```python
from build123d import *


with BuildPart() as part:
    # Croquis1 → Revolución1 (revolve)
    with BuildSketch(Plane.XY):
        with BuildLine():
            Line((5, 0), (15, 0))
            ThreePointArc((15, 0), (17.5, 2.5), (15, 5))
            Line((15, 5), (17, 9.999396685))
            ThreePointArc((17, 9.999396685), (25.700254064, 18.050962315), (18.873239437, 27.741885964))
            ThreePointArc((18.873239437, 27.741885964), (9.503923477, 29.433465482), (0, 30))
            Line((0, 30), (0, 10))
            Line((0, 10), (5, 10))
            Line((5, 10), (5, 0))
        make_face()
    revolve(axis=Axis((0, -10.165252064, 0), (0, 1, 0)))


solid = part.part
```
Geometry check sheet. Reference: the model listing, model coordinates, mm. A direction names the side the tool comes from. Give positions to 0.01 mm unless a question says otherwise; leave off trailing zeros. Write each loop counter-clockwise with the first axis right and the second up, starting at its lowest first coordinate (ties: lowest second). Pieces come first, ordered by that corner, then holes. Notation, with made-up numbers: (27.25, 88) - (59.25, 88) arc R22 cw to (59.25, 126) - close; hole circle Ø6 at (29.25, 32.5). An arc over 180 degrees is marked (long way). Use a Markdown table: item, result.
Q1. Section check D-D, the plane y = 18.5. Enter the section's corners in (x, z).
Computed:
| item | result |
|---|---|
| outline | circle Ø51.47 at (0, 0) |
Q2. Thickness scan on L1, parallel to Z at x = 0, y = 4; L2, parallel to X at y = 8, z = 0; L3, parallel to Y at x = -0.5, z = -16.5. Record the ranges inside material, lowest first. Write a range as [from, to].
Computed:
| item | result |
|---|---|
| L1 | z = [-17, -5], [5, 17] |
| L2 | x = [-16.2, -5], [5, 16.2] |
| L3 | y = [0.51, 4.49], [8.77, 28.28] |
Q3. Section check B-B, the plane x = 0. Enter the section's corners in (y, z).
Computed:
| item | result |
|---|---|
| outline | (0, -15) arc R2.5 ccw to (5, -15) - (10, -17) arc R9 ccw to (27.74, -18.87) arc R80 ccw to (27.74, 18.87) arc R9 ccw to (10, 17) - (5, 15) arc R2.5 ccw to (0, 15) - (0, 5) - (10, 5) - (10, -5) - (0, -5) - close |
Q4. Section check A-A, the plane z = 0. Enter the section's corners in (x, y).
Computed:
| item | result |
|---|---|
| outline | (-18.87, 27.74) arc R9 ccw to (-17, 10) - (-15, 5) arc R2.5 ccw to (-15, 0) - (-5, 0) - (-5, 10) - (5, 10) - (5, 0) - (15, 0) arc R2.5 ccw to (15, 5) - (17, 10) arc R9 ccw to (18.87, 27.74) arc R80 ccw to start |
Q5. Draft check along Z on faces 3 (the face through (4, 0, -4)), 4 (the face through (-1.08, 4.93, 4.88)). Enter one of: pulls with the +Z half, pulls with the -Z half, needs draft (parallel to the pull), parting line crosses it, or undercut.
Computed:
| item | result |
|---|---|
| face 3 | needs draft |
| face 4 | undercut |
Q6. Go/stop test with flat-tipped pins: P1, Ø4, axis at y = 10.5, z = 12, coming from the -X side; P2, Ø12, axis at x = -16.5, z = -20, coming from the +Y side; P3, Ø8, axis at x = -1, y = 15, coming from the -Z side; P4, Ø11.5, axis at x = 0, z = 0, coming from the -Y side. Record where each tip stops, or that it passes through.
Computed:
| item | result |
|---|---|
| P1 | stops at x = -19.86 |
| P2 | stops at y = 27.42 |
| P3 | stops at z = -25.75 |
| P4 | stops at y = 0 |
Q7. Set-up check for faces 1 (the face through (0, 10, 0)), 2 (the face through (-3.279, 5.313, 14.765)): record each of +Z, -Z, +X, -X, +Y, -Y from which the full face is reachable in a straight line by a thin tool's end or side.
Computed:
| item | result |
|---|---|
| face 1 | -Y |
| face 2 | none |
Q8. Section check C-C, the plane y = 7.25. Enter the section's corners in (x, z), then the cut area to 3 significant figures.
Computed:
| item | result |
|---|---|
| outline | circle Ø31.8 at (0, 0); hole circle Ø10 at (0, 0) |
| area | 716 mm² |
